Check sheet for the drawn part. Datum: minimum x, y, z corner. Units: mm. A direction names the side the tool comes from. Round coordinates to 2 decimals unless told otherwise and drop trailing zeros. Order: outer loops, then holes, each group sorted by start corner. A loop starts at its lowest first (then second) coordinate and runs counter-clockwise, first axis right, second up. Notation, with made-up numbers: (40, 49.25) - (72, 49.25) arc R13 cw to (72, 55.25) - close; hole circle Ø1 at (84, 11). An arc over 180 degrees is marked (long way). Write each question's results on one line, items separated by ' | '.
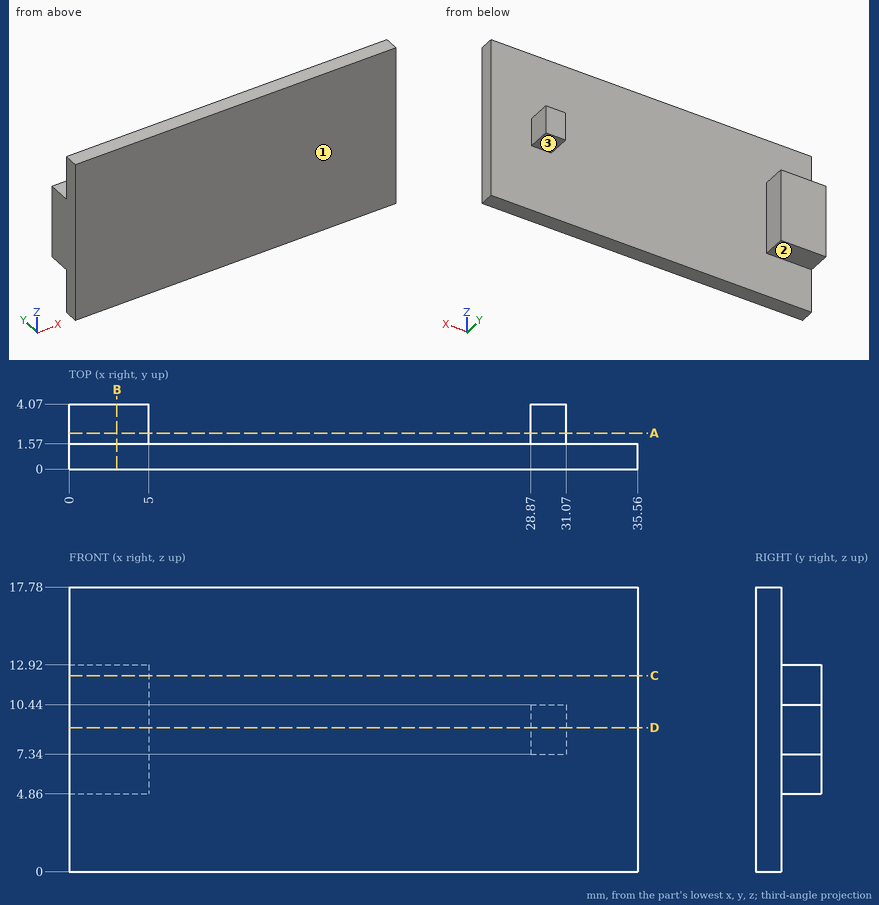
(1) Section check B-B (x = 3). Record the cut outline in (y, z).
Answers follow:
outline: (0, 0) - (1.57, 0) - (1.57, 4.86) - (4.07, 4.86) - (4.07, 12.92) - (1.57, 12.92) - (1.57, 17.78) - (0, 17.78) - close
(2) Material ranges on line 1 (X direction, y = 1.9, z = 8.75); line 2 (Z direction, x = 3, y = 3); line 3 (X direction, y = 2.45, z = 5), recorded low to high.
Answers follow:
line 1: 0 to 5, 28.87 to 31.07 | line 2: 4.86 to 12.92 | line 3: 0 to 5
(3) Section check C-C (z = 12.25). Record the cut outline in (x, y), then the cut area to 3 significant figures.
Answers follow:
outline: (0, 0) - (35.56, 0) - (35.56, 1.57) - (5, 1.57) - (5, 4.07) - (0, 4.07) - close | area: 68.3 mm²
(4) Section check D-D (z = 9). Record the cut outline in (x, y), then the cut area to 3 significant figures.
Answers follow:
outline: (0, 0) - (35.56, 0) - (35.56, 1.57) - (31.07, 1.57) - (31.07, 4.07) - (28.87, 4.07) - (28.87, 1.57) - (5, 1.57) - (5, 4.07) - (0, 4.07) - close | area: 73.8 mm²
(5) Section check A-A (y = 2.25). Record the cut outline in (x, z).
Answers follow:
outline: (0, 4.86) - (5, 4.86) - (5, 12.92) - (0, 12.92) - close; (28.87, 7.34) - (31.07, 7.34) - (31.07, 10.44) - (28.87, 10.44) - close
(6) Depth check by flat-ended pin: pin 1 Ø0.7 at (x, y) = (30, 2.5) entering from -Z; pin 2 Ø5.5 at (x, z) = (12, 10.5) entering from +Y; pin 3 Ø0.8 at (y, z) = (2, 8) entering from +X; pin 4 Ø2 at (x, y) = (13, 3) entering from -Z. Enter the tip coordinate at first touch or a pass-through.
Answers follow:
pin 1: z = 7.34 | pin 2: y = 1.57 | pin 3: x = 31.07 | pin 4: through
(7) Access from +Z, -Z, +X, -X, +Y, -Y to the whole of each face (thin tool, end or side, straight path). Record for the marked faces 1, 2 and 3.
Answers follow:
face 1: +Z, -Z, +X, -X, -Y | face 2: -Z, +X, -X, +Y | face 3: -Z, +X, +Y
